```python
from build123d import *

# Parameters (mm, degrees)
SKETCH1_W           = 37.2872
SKETCH1_H           = 60.325
BOSS_EXTRUDE1_DEPTH = 28.575
FILLET1_R           = 4.7625
SHELL1_T            = -1.5875


with BuildPart() as part:
    # Sketch1 → Boss-Extrude1 (new body)
    with BuildSketch(Plane(origin=(0, 0, 0), x_dir=(1, 0, 0), z_dir=(0, 1, 0))):
        Rectangle(SKETCH1_W, SKETCH1_H)
    extrude(amount=BOSS_EXTRUDE1_DEPTH)

    # Fillet1
    fillet1_edges = [part.edges().sort_by_distance(p)[0] for p in [
        (0, 28.575, 30.1625),
        (18.6436, 28.575, 0),
        (0, 28.575, -30.1625),
        (18.6436, 14.2875, 30.1625),
        (18.6436, 14.2875, -30.1625),
    ]]
    fillet(fillet1_edges, radius=FILLET1_R)

    # Shell1
    shell1_openings = [part.faces().sort_by_distance(p)[0] for p in [
        (-0.076414213, 0, 0),
        (-18.6436, 14.212396054, 0),
    ]]
    offset(amount=SHELL1_T, openings=shell1_openings, kind=Kind.INTERSECTION)


solid = part.part
```
Part model, mm, in its own coordinate system. A direction names the side the tool comes from. Coordinates: 2 decimals unless noted, no trailing zeros. Return JSON: item names as keys, results as strings. Group by question number.
Item 1: Which spindle directions (+Z, -Z, +X, -X, +Y, -Y) get a long thin tool onto all of the face, cutting with end or side? Do faces 1 (the face through (-3, 26.988, 0)), 2 (the face through (-3, 28.575, 0)). Say none if no direction does.
Item 2: Pull direction Z, two halves, no side cores. Call faces 3 (the face through (-3, 12, 30.162)), 4 (the face through (16.1, 12.07, 27.67)), 5 (the face through (18.644, 12, 0)): pulls with the +Z half, pulls with the -Z half, needs draft (parallel to the pull), parting line crosses it, or undercut.
Item 3: Pin check, flat tips, straight feed: pin 1 (5 mm diameter, centred on x = 0, z = -3, fed in from -Y); pin 2 (2 mm diameter, centred on y = 11.5, z = 4, fed in from -X). Stop position of each tip, or through.
Item 4: Drill centre lines: probe 1 along Z at (x, y) = (7, 14.5) (1 decimal); probe 2 along X at (y, z) = (21.5, 10.5); probe 3 along Y at (x, z) = (3.5, 0.5) (1 decimal). Where is each one in solid material? Low to high. Write a range as from..to.
Check values:
{
 "1": {"face 1": "-X, -Y", "face 2": "+Z, -Z, +X, -X, +Y"},
 "2": {"face 3": "pulls with the +Z half", "face 4": "undercut", "face 5": "needs draft"},
 "3": {"pin 1": "stops at y = 26.99", "pin 2": "stops at x = 17.06"},
 "4": {"probe 1": "z = -30.2..-28.6, 28.6..30.2", "probe 2": "x = 17.06..18.64", "probe 3": "y = 27..28.6"}
}
